Work out the finished part from the listing and answer in its coordinate system (mm). Coordinates: 2 decimals unless noted, no trailing zeros. Order: outer loops, then holes, each group sorted by start corner. A loop starts at its lowest first (then second) coordinate and runs counter-clockwise, first axis right, second up. Notation, with made-up numbers: M 32,77 L 59,77 A17 cw 59,103 Z; hole C 52.5,-28.75 d2. An arc over 180 degrees is marked long. Use a Markdown table: item, result.
from build123d import *

# Parameters (mm, degrees)
ESBO_O1_W                = 250
ESBO_O1_H                = 250
RESSALTO_EXTRUS_O1_DEPTH = 5
ESBO_O2_R                = 3.5
CORTE_EXTRUS_O1_DEPTH    = 177.847391838
ESBO_O3_W                = 121
ESBO_O3_H                = 121
CORTE_EXTRUS_O2_DEPTH    = 177.847391838


with BuildPart() as part:
    # Esboço1 → Ressalto-extrusão1 (new body)
    with BuildSketch(Plane.XY):
        Rectangle(ESBO_O1_W, ESBO_O1_H)
    extrude(amount=RESSALTO_EXTRUS_O1_DEPTH)

    # Esboço2 → Corte-extrusão1 (cut, through all)
    with BuildSketch(Plane.XY.offset(5)):
        with Locations((-117.5, 117.5)):
            Circle(ESBO_O2_R)
        with Locations(Location((117.5, 117.5, 0), (0, 0, 180))):
            Circle(ESBO_O2_R)
        with Locations(Location((-117.5, -117.5, 0), (0, 0, 180))):
            Circle(ESBO_O2_R)
        with Locations((117.5, -117.5)):
            Circle(ESBO_O2_R)
    extrude(amount=-CORTE_EXTRUS_O1_DEPTH, mode=Mode.SUBTRACT)

    # Esboço3 → Corte-extrusão2 (cut, through all)
    with BuildSketch(Plane.XY.offset(5)):
        Rectangle(ESBO_O3_W, ESBO_O3_H)
    extrude(amount=-CORTE_EXTRUS_O2_DEPTH, mode=Mode.SUBTRACT)


solid = part.part
(1) A cutting plane is placed at C-C (z = 3.9). Determine the outline of the cut face in (x, y).
Conclusion:
| item | result |
|---|---|
| outline | M -125,-125 L 125,-125 L 125,125 L -125,125 Z; hole C -117.5,-117.5 d7; hole C -117.5,117.5 d7; hole M -60.5,-60.5 L 60.5,-60.5 L 60.5,60.5 L -60.5,60.5 Z; hole C 117.5,-117.5 d7; hole C 117.5,117.5 d7 |
(2) Determine the mould class of faces 1 (the flat face through (-2, 85, 0)), 2 (the cylindrical face through (-114.267, 116.159, 2.535)) for opening direction Y: pulls with the +Y half, pulls with the -Y half, needs draft (parallel to the pull), parting line crosses it, or undercut.
Conclusion:
| item | result |
|---|---|
| face 1 | needs draft |
| face 2 | undercut |
(3) A cutting plane is placed at A-A (y = -44.5). Determine the outline of the cut face in (x, z), then the cut area to 3 significant figures.
Conclusion:
| item | result |
|---|---|
| outline | M -125,0 L -60.5,0 L -60.5,5 L -125,5 Z; M 60.5,0 L 125,0 L 125,5 L 60.5,5 Z |
| area | 645 mm2 |
(4) Straight lines are drawn through the part: L1, parallel to Y at x = 117.5, z = 2.45; L2, parallel to X at y = -42, z = 1.45. For each, find the intervals that lie inside material, in ascending order.
Conclusion:
| item | result |
|---|---|
| L1 | -125 to -121, -114 to 114, 121 to 125 |
| L2 | -125 to -60.5, 60.5 to 125 |
(5) Given P1, Ø5.5, axis at x = -117.5, y = -117.5, coming from the +Z side, flat-ended and moving along its own axis, determine where the tip first touches the part or whether it passes through.
Conclusion:
| item | result |
|---|---|
| P1 | through |
(6) A cutting plane is placed at B-B (x = 117.5). Determine the outline of the cut face in (y, z), then the cut area to 3 significant figures.
Conclusion:
| item | result |
|---|---|
| outline | M -125,0 L -121,0 L -121,5 L -125,5 Z; M -114,0 L 114,0 L 114,5 L -114,5 Z; M 121,0 L 125,0 L 125,5 L 121,5 Z |
| area | 1,180 mm2 |
